Geometry check sheet. Reference: the model listing, model coordinates, mm. Face numbers are marked on the shaded views. A direction names the side the tool comes from. Round coordinates to 2 decimals unless told otherwise and drop trailing zeros. Order: outer loops, then holes, each group sorted by start corner. A loop starts at its lowest first (then second) coordinate and runs counter-clockwise, first axis right, second up. Notation, with made-up numbers: (83, -1.75) - (121, -1.75) arc R25 cw to (121, 35.25) - close; hole circle Ø7 at (-16.5, 29.5). An arc over 180 degrees is marked (long way). Answer as CSV lines item,"result". Start each with the question number.
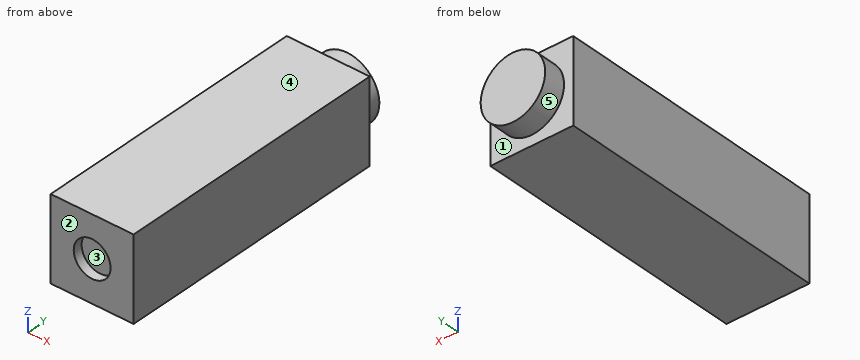
```python
from build123d import *

# Parameters (mm, degrees)
SKETCH1_W           = 4.5
SKETCH1_H           = 4.5
BOSS_EXTRUDE1_DEPTH = 15
SKETCH2_R           = 1
CUT_EXTRUDE1_DEPTH  = 0.5
SKETCH4_R           = 1.75
BOSS_EXTRUDE2_DEPTH = 1.2


with BuildPart() as part:
    # Sketch1 → Boss-Extrude1 (new body)
    with BuildSketch(Plane(origin=(0, 0, 0), x_dir=(1, 0, 0), z_dir=(0, 1, 0))):
        Rectangle(SKETCH1_W, SKETCH1_H)
    extrude(amount=BOSS_EXTRUDE1_DEPTH)

    # Sketch2 → Cut-Extrude1 (cut)
    with BuildSketch(Plane.XZ):
        with Locations(Location((0, 0, 0), (0, 0, 270))):
            Circle(SKETCH2_R)
    extrude(amount=-CUT_EXTRUDE1_DEPTH, mode=Mode.SUBTRACT)

    # Sketch4 → Boss-Extrude2 (add)
    with BuildSketch(Plane(origin=(0, 15, 0), x_dir=(1, 0, 0), z_dir=(0, 1, 0))):
        with Locations(Location((0, -0.04771887, 0), (0, 0, 270))):
            Circle(SKETCH4_R)
    extrude(amount=BOSS_EXTRUDE2_DEPTH)


solid = part.part
```
1. Thickness scan on probe 1 along X at (y, z) = (0.45, 0); probe 2 along Y at (x, z) = (1.1, -2.05); probe 3 along Y at (x, z) = (0.85, -0.1). Record the ranges inside material, lowest first.
2. Section check A-A on x = -0.2. Record the boundary of the cut face in (y, z), plus the area to 3 significant figures.
3. Access from +Z, -Z, +X, -X, +Y, -Y to the whole of each face (thin tool, end or side, straight path). Record for the marked faces 1 and 2.
4. Section check B-B on z = 0. Record the boundary of the cut face in (x, y).
5. Section check C-C on y = 15.25. Record the boundary of the cut face in (x, z), plus the area to 3 significant figures.
6. Section check D-D on x = -1.15. Record the boundary of the cut face in (y, z).
7. Draft check along X on the marked faces 3, 4 and 5. Enter one of: released by +X, released by -X, zero draft, split by the parting line, or undercut.
Numbers:
1,probe 1,"x = -2.25 to -1, 1 to 2.25"
1,probe 2,"y = 0 to 15"
1,probe 3,"y = 0.5 to 16.2"
2,outline,"(0, -2.25) - (15, -2.25) - (15, -1.69) - (16.2, -1.69) - (16.2, 1.79) - (15, 1.79) - (15, 2.25) - (0, 2.25) - (0, 0.98) - (0.5, 0.98) - (0.5, -0.98) - (0, -0.98) - close"
2,area,"70.7 mm2"
3,face 1,"+Y"
3,face 2,"+Z, -Z, +X, -X, -Y"
4,outline,"(-2.25, 0) - (-1, 0) - (-1, 0.5) - (1, 0.5) - (1, 0) - (2.25, 0) - (2.25, 15) - (1.75, 15) - (1.75, 16.2) - (-1.75, 16.2) - (-1.75, 15) - (-2.25, 15) - close"
5,outline,"circle Ø3.5 at (0, 0.05)"
5,area,"9.62 mm2"
6,outline,"(0, -2.25) - (15, -2.25) - (15, -1.27) - (16.2, -1.27) - (16.2, 1.37) - (15, 1.37) - (15, 2.25) - (0, 2.25) - close"
7,face 3,"undercut"
7,face 4,"zero draft"
7,face 5,"split by the parting line"
